Could you check a few things on this model? Use its own coordinates, in mm. Coordinates: 2 decimals unless noted, no trailing zeros. One line per item, written item: value. Start each with the question number.
(1) I'm going to push flat-ended pins straight in: P1, Ø1.2, axis at x = 154, z = 5.5, coming from the +Y side; P2, Ø5, axis at x = 62, y = -5.5, coming from the -Z side. Where does each tip first touch, or does it pass through?
(2) If I drill on line 1 along Y through (x, z) = (22.5, 6.25), over which ranges is the centre line in solid material (lowest first)? Write a range as from..to.
(3) If we section it at A-A on y = -0.25: Count the separate pieces of the cut face and the enclosed holes in it, then the cut area to 3 significant figures.
```python
from build123d import *

# Parameters (mm, degrees)
BOSS_EXTRU_1_DEPTH         = 10
R_P_TITION_LIN_AIRE1_COUNT = 30
R_P_TITION_LIN_AIRE1_PITCH = 6.283


with BuildPart() as part:
    # Esquisse1 → Boss.-Extru.1 (new body)
    with BuildSketch(Plane.XY):
        Polygon((0.831079968, 2), (2.377953464, -2.25), (3.905046536, -2.25), (3.905046536, -12.25), (-2.377953464, -12.25), (-2.377953464, -2.25), (-0.831079968, 2), align=None)
    boss_extru_1 = extrude(amount=BOSS_EXTRU_1_DEPTH)

    # Répétition linéaire1: Boss.-Extru.1 ×30
    with Locations(*[(i * R_P_TITION_LIN_AIRE1_PITCH, 0, 0) for i in range(1, R_P_TITION_LIN_AIRE1_COUNT)]):
        add(boss_extru_1)


solid = part.part
```
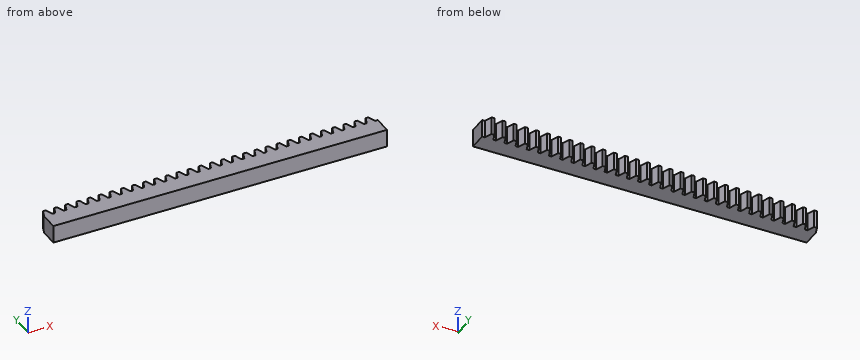
Values:
1. P1: stops at y = -2.25
1. P2: stops at z = 0
2. line 1: y = -12.25..-2.25
3. separate pieces: 30
3. enclosed holes: 0
3. area: 990 mm2
